Work out the finished part from the listing and answer in its coordinate system (mm). A direction names the side the tool comes from. Coordinates: 2 decimals unless noted, no trailing zeros. Write each loop counter-clockwise with the first axis right and the second up, starting at its lowest first coordinate (ties: lowest second). Pieces come first, ordered by that corner, then holes. Notation, with made-up numbers: (18, -2) - (77, -2) arc R13 ccw to (77, 20) - close; hole circle Ø1 at (36, -39). An arc over 180 degrees is marked (long way). Use one line per item in the form item = value. Start each with the question number.
Item 1: A cutting plane is placed at B-B (z = 6). Write down the section's boundary in (x, y).
Item 2: A cutting plane is placed at D-D (z = 26). Write down the section's boundary in (x, y) (3 decimals), then the cut area to 3 significant figures.
Item 3: A cutting plane is placed at A-A (x = 0). Write down the section's boundary in (y, z) (3 decimals), then the cut area to 3 significant figures.
Item 4: Consider probe 1 along X at (y, z) = (-10, 6); probe 2 along Y at (x, z) = (0, 19); probe 3 along Y at (x, z) = (-5, 19). Determine where each line is inside the solid, lowest interval first.
Item 5: Determine the mould class of faces 1 (the flat face through (-8, -17, 20)), 2 (the flat face through (0, -20, 32)), 3 (the cylindrical face through (0, -2, 18)) for opening direction X: released by +X, released by -X, zero draft, split by the parting line, or undercut.
Item 6: For faces 4 (the flat face through (-6, 0, 16)), 5 (the flat face through (0, -12, 6)), 6 (the flat face through (6, -5, 20)), 7 (the flat face through (0, -12, 22)), determine the directions among +Z, -Z, +X, -X, +Y, -Y from which every point of the face is accessible in a straight line to the end or side of a thin tool.
Item 7: A cutting plane is placed at C-C (y = 5). Write down the section's boundary in (x, z) (3 decimals).
Item 8: Given pin 1 (2 mm diameter, centred on x = 6.5, y = -3.5, fed in from +Z); pin 2 (8 mm diameter, centred on x = 3.5, z = 23, fed in from +Y); pin 3 (0.8 mm diameter, centred on x = -1.5, y = 11, fed in from +Z), each flat-ended and moving along its own axis, determine where each tip first touches the part or whether it passes through.
from build123d import *

# Parameters (mm, degrees)
SKETCH1_W                                   = 44
SKETCH1_H                                   = 24
CROSSHEAD_BASE_DEPTH                        = 12
SHOE_UPRISER_START                          = 12
SKETCH2_W                                   = 8
SKETCH2_H                                   = 24
SHOE_UPRISER_DEPTH                          = 11
ADAPTER_BRIDGE_START                        = 12
SKETCH3_W                                   = 16
SKETCH3_H                                   = 28
ADAPTER_BRIDGE_DEPTH                        = 8
THREADED_ROD_ADAPTER_START                  = 20
SKETCH4_W                                   = 16
SKETCH4_H                                   = 16
THREADED_ROD_ADAPTER_DEPTH                  = 12
TWO_BRONZE_BUSH_HOUSINGS_DEPTH              = 48.874836814
TWO_BRONZE_BUSH_HOUSINGS_DEPTH_BACK         = 48.874836814
SKETCH5_R                                   = 5
QUARTER20_ADAPTER_MAJOR_ENVELOPE_DEPTH      = 48.874836814
QUARTER20_ADAPTER_MAJOR_ENVELOPE_DEPTH_BACK = 48.874836814
SKETCH6_R                                   = 3.175
SKETCH7_R                                   = 2
M4_SHOE_THREAD_MAJOR_ENVELOPE_DEPTH         = 11
CROSS_SLOT_BOTTOM_CLEARANCE_DEPTH           = 48.874836873
CROSS_SLOT_BOTTOM_CLEARANCE_DEPTH_BACK      = 48.874836873
SKETCH8_W                                   = 5.5
SKETCH8_H                                   = 2.5
SKETCH8_H_2                                 = 3


with BuildPart() as part:
    # Sketch1 → Crosshead_Base (new body)
    with BuildSketch(Plane.XY):
        Rectangle(SKETCH1_W, SKETCH1_H)
    extrude(amount=CROSSHEAD_BASE_DEPTH)

    # Sketch2 → Shoe_Upriser (add)
    with BuildSketch(Plane.XY.offset(SHOE_UPRISER_START)):
        Rectangle(SKETCH2_W, SKETCH2_H)
    extrude(amount=SHOE_UPRISER_DEPTH)

    # Sketch3 → Adapter_Bridge (add)
    with BuildSketch(Plane.XY.offset(ADAPTER_BRIDGE_START)):
        with Locations((0, -14)):
            Rectangle(SKETCH3_W, SKETCH3_H)
    extrude(amount=ADAPTER_BRIDGE_DEPTH)

    # Sketch4 → Threaded_Rod_Adapter (add)
    with BuildSketch(Plane.XY.offset(THREADED_ROD_ADAPTER_START)):
        with Locations((0, -20)):
            Rectangle(SKETCH4_W, SKETCH4_H)
    extrude(amount=THREADED_ROD_ADAPTER_DEPTH)

    # Sketch5 → Two_Bronze_Bush_Housings (cut, two sides: drawn at the far end of the back side and taken through both)
    with BuildSketch(Plane(origin=(0, 0, 0), x_dir=(1, 0, 0), z_dir=(0, 1, 0)).offset(-TWO_BRONZE_BUSH_HOUSINGS_DEPTH_BACK)):
        with Locations(Location((-14, -6, 0), (0, 0, 270))):
            Circle(SKETCH5_R)
        with Locations(Location((14, -6, 0), (0, 0, 270))):
            Circle(SKETCH5_R)
    extrude(amount=TWO_BRONZE_BUSH_HOUSINGS_DEPTH + TWO_BRONZE_BUSH_HOUSINGS_DEPTH_BACK, mode=Mode.SUBTRACT)

    # Sketch6 → Quarter20_Adapter_Major_Envelope (cut, two sides: drawn at the far end of the back side and taken through both)
    with BuildSketch(Plane(origin=(0, 0, 0), x_dir=(1, 0, 0), z_dir=(0, 1, 0)).offset(-QUARTER20_ADAPTER_MAJOR_ENVELOPE_DEPTH_BACK)):
        with Locations(Location((0, -26, 0), (0, 0, 270))):
            Circle(SKETCH6_R)
    extrude(amount=QUARTER20_ADAPTER_MAJOR_ENVELOPE_DEPTH + QUARTER20_ADAPTER_MAJOR_ENVELOPE_DEPTH_BACK, mode=Mode.SUBTRACT)

    # Sketch7 → M4_Shoe_Thread_Major_Envelope (cut)
    with BuildSketch(Plane.XY.offset(23)):
        Circle(SKETCH7_R)
    extrude(amount=-M4_SHOE_THREAD_MAJOR_ENVELOPE_DEPTH, mode=Mode.SUBTRACT)

    # Sketch8 → Cross_Slot_Bottom_Clearance (cut, two sides: drawn at the far end of the back side and taken through both)
    with BuildSketch(Plane(origin=(0, 0, 0), x_dir=(0, 0, -1), z_dir=(1, 0, 0)).offset(-CROSS_SLOT_BOTTOM_CLEARANCE_DEPTH_BACK)):
        with Locations((-20.75, -10.75)):
            Rectangle(SKETCH8_W, SKETCH8_H)
        with Locations((-20.75, 11)):
            Rectangle(SKETCH8_W, SKETCH8_H_2)
    extrude(amount=CROSS_SLOT_BOTTOM_CLEARANCE_DEPTH + CROSS_SLOT_BOTTOM_CLEARANCE_DEPTH_BACK, mode=Mode.SUBTRACT)


solid = part.part
Answer:
q1.outline = (-22, -12) - (-19, -12) - (-19, 12) - (-22, 12) - close; (-9, -12) - (9, -12) - (9, 12) - (-9, 12) - close; (19, -12) - (22, -12) - (22, 12) - (19, 12) - close
q2.outline = (-8, -28) - (-3.175, -28) - (-3.175, -12) - (-8, -12) - close; (3.175, -28) - (8, -28) - (8, -12) - (3.175, -12) - close
q2.area = 154 mm²
q3.outline = (-28, 12) - (-12, 12) - (-12, 0) - (12, 0) - (12, 18) - (9.5, 18) - (9.5, 22.825) - (2, 22.825) - (2, 12) - (-2, 12) - (-2, 22.825) - (-9.5, 22.825) - (-9.5, 18) - (-12, 18) - (-12, 22.825) - (-28, 22.825) - close; (-28, 29.175) - (-12, 29.175) - (-12, 32) - (-28, 32) - close
q3.area = 699 mm²
q4.probe_1 = -22 to -19, -9 to 9, 19 to 22
q4.probe_2 = -28 to -12, -9.5 to -2, 2 to 9.5
q4.probe_3 = -28 to -12, -9.5 to 0
q5.face_1 = released by -X
q5.face_2 = zero draft
q5.face_3 = undercut
q6.face_4 = +Z, -X, +Y
q6.face_5 = -Z, +X, -X, -Y
q6.face_6 = +Z, +X, +Y
q6.face_7 = +Z, +X, -X
q7.outline = (-22, 0) - (22, 0) - (22, 12) - (4, 12) - (4, 23) - (1.04, 23) arc R3.175 cw to (-1.04, 23) - (-4, 23) - (-4, 12) - (-22, 12) - close; hole circle Ø10 at (-14, 6); hole circle Ø10 at (14, 6)
q8.pin_1 = 20
q8.pin_2 = 9.5
q8.pin_3 = 18
